Here's how the part is built. I have some questions about the finished solid (model axes, mm). Give positions to 0.01 mm unless a question says otherwise; leave off trailing zeros. Loops run counter-clockwise (first coordinate to the right, second up) from the corner with the lowest first, then second, coordinate; pieces in that order, holes last.
Q1. Will these pins go through, and if not, where does the flat tip stop? P1, Ø0.9, axis at y = 1, z = -70.5, coming from the -X side; P2, Ø0.9, axis at y = 1, z = -17, coming from the +X side; P3, Ø0.9, axis at x = 160, y = 1.5, coming from the -Z side.
Q2. If we section it at A-A (z = -70): Please give me the cut outline in (x, y), plus the area to 3 significant figures.
Q3. I need wall thicknesses on line 1 (X direction, y = 2.1, z = -72.5); line 2 (X direction, y = 1.55, z = -55.5); line 3 (X direction, y = 2, z = -16). Which ranges of each line are inside material? Lowest first, please.
Q4. If we section it at B-B (x = 79): Please give me the cut outline in (y, z).
from build123d import *

# Parameters (mm, degrees)
SKETCH1_W           = 560
SKETCH1_H           = 75
BOSS_EXTRUDE1_DEPTH = 3
SKETCH2_W           = 50
SKETCH2_H           = 31
SKETCH2_W_2         = 25
CUT_EXTRUDE2_DEPTH  = 3
SKETCH3_W           = 20
SKETCH3_H           = 3
CUT_EXTRUDE3_DEPTH  = 3
SKETCH7_W           = 3
SKETCH7_H           = 15
SKETCH7_H_2         = 11
SKETCH7_H_3         = 18
CUT_EXTRUDE8_DEPTH  = 10


with BuildPart() as part:
    # Sketch1 → Boss-Extrude1 (new body)
    with BuildSketch(Plane(origin=(0, 0, 0), x_dir=(1, 0, 0), z_dir=(0, 1, 0))):
        with Locations((103.055832565, 47.017453799)):
            Rectangle(SKETCH1_W, SKETCH1_H)
    extrude(amount=BOSS_EXTRUDE1_DEPTH)

    # Sketch2 → Cut-Extrude2 (cut)
    with BuildSketch(Plane(origin=(0, 3, 0), x_dir=(1, 0, 0), z_dir=(0, 1, 0))):
        with Locations((-1.944167435, 69.017453799)):
            Rectangle(SKETCH2_W, SKETCH2_H)
        with Locations((75.555832565, 69.017453799)):
            Rectangle(SKETCH2_W_2, SKETCH2_H)
        with Locations((163.055832565, 69.017453799)):
            Rectangle(SKETCH2_W, SKETCH2_H)
        with Locations((245.555832565, 69.017453799)):
            Rectangle(SKETCH2_W_2, SKETCH2_H)
    extrude(amount=-CUT_EXTRUDE2_DEPTH, mode=Mode.SUBTRACT)

    # Sketch3 → Cut-Extrude3 (cut)
    with BuildSketch(Plane(origin=(0, 3, 0), x_dir=(1, 0, 0), z_dir=(0, 1, 0))):
        with Locations((-166.944167435, 83.017453799)):
            Rectangle(SKETCH3_W, SKETCH3_H)
    extrude(amount=-CUT_EXTRUDE3_DEPTH, mode=Mode.SUBTRACT)

    # Sketch7 → Cut-Extrude8 (cut)
    with BuildSketch(Plane(origin=(0, 3, 0), x_dir=(1, 0, 0), z_dir=(0, 1, 0))):
        with Locations((-175.444167435, 17.017453799)):
            Rectangle(SKETCH7_W, SKETCH7_H)
        with Locations((-175.444167435, 44.017453799)):
            Rectangle(SKETCH7_W, SKETCH7_H_2)
        with Locations((-175.444167435, 72.517453799)):
            Rectangle(SKETCH7_W, SKETCH7_H_3)
        with Locations((381.555832565, 17.017453799)):
            Rectangle(SKETCH7_W, SKETCH7_H)
        with Locations((381.555832565, 44.017453799)):
            Rectangle(SKETCH7_W, SKETCH7_H_2)
        with Locations((381.555832565, 72.517453799)):
            Rectangle(SKETCH7_W, SKETCH7_H_3)
        Polygon((383.055832565, 81.517453799), (383.055832565, 84.517453799), (363.055832565, 84.517453799), (363.055832565, 81.517453799), (380.055832565, 81.517453799), align=None)
    extrude(amount=-CUT_EXTRUDE8_DEPTH, mode=Mode.SUBTRACT)


solid = part.part
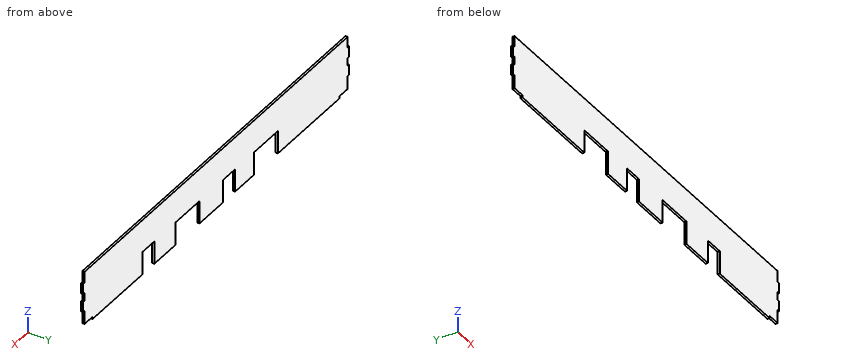
Check sheet entries:
1. P1: stops at x = -173.94
1. P2: stops at x = 380.06
1. P3: stops at z = -53.52
2. outline: (-173.94, 0) - (-26.94, 0) - (-26.94, 3) - (-173.94, 3) - close; (23.06, 0) - (63.06, 0) - (63.06, 3) - (23.06, 3) - close; (88.06, 0) - (138.06, 0) - (138.06, 3) - (88.06, 3) - close; (188.06, 0) - (233.06, 0) - (233.06, 3) - (188.06, 3) - close; (258.06, 0) - (380.06, 0) - (380.06, 3) - (258.06, 3) - close
2. area: 1,210 mm2
3. line 1: x = -173.94 to -26.94, 23.06 to 63.06, 88.06 to 138.06, 188.06 to 233.06, 258.06 to 380.06
3. line 2: x = -176.94 to -26.94, 23.06 to 63.06, 88.06 to 138.06, 188.06 to 233.06, 258.06 to 383.06
3. line 3: x = -173.94 to 380.06
4. outline: (0, -53.52) - (3, -53.52) - (3, -9.52) - (0, -9.52) - close
